Source: CAD feature listing. Evaluate the final solid. Frame: model axes, mm. A direction names the side the tool comes from. Round coordinates to 2 decimals unless told otherwise and drop trailing zeros. Order: outer loops, then holes, each group sorted by start corner. A loop starts at its lowest first (then second) coordinate and runs counter-clockwise, first axis right, second up. Notation, with made-up numbers: (61, 83) -> (92, 83) arc R18 cw to (92, 108) -> close; hole circle Ø4 at (88, 20). An arc over 180 degrees is marked (long way). Use a Markdown table: item, result. Add a question column.
```python
from build123d import *

# Parameters (mm, degrees)
AUFSATZ_LINEAR_AUSTRAGEN1_DEPTH             = 20
AUFSATZ_LINEAR_AUSTRAGEN2_REACH             = 50.332
AUFSATZ_LINEAR_AUSTRAGEN2_DIRECTION_2_REACH = 50.332
SKIZZE2_R                                   = 2.3
SCHNITT_LINEAR_AUSTRAGEN1_DEPTH             = 20
SKIZZE4_R                                   = 4.2
SCHNITT_LINEAR_AUSTRAGEN2_DEPTH             = 20
VERRUNDUNG1_R                               = 0.75
VERRUNDUNG2_R                               = 4
SKIZZE5_R                                   = 1.7499999999999998
SCHNITT_LINEAR_AUSTRAGEN3_DEPTH             = 20
FASE1_SIZE                                  = 0.5


with BuildPart() as part:
    # Skizze1 → Aufsatz-Linear austragen1 (new body)
    with BuildSketch(Plane.XY):
        Polygon((-11, 0), (11, 0), (21.999999999999947, 19.052558883257674), (10.999999999999858, 38.10511776651528), (-10.999999999999858, 38.10511776651528), (-21.999999999999947, 19.052558883257674), align=None)
        Polygon((0, 7), (6.958548115672608, 7), (13.917096231345187, 19.052558883257657), (6.958548115672503, 31.105117766515278), (-6.958548115672498, 31.105117766515278), (-13.917096231345184, 19.05255888325765), (-6.958548115672604, 7), align=None, mode=Mode.SUBTRACT)
    extrude(amount=AUFSATZ_LINEAR_AUSTRAGEN1_DEPTH)

    # Aufsatz-Linear austragen2: up to this plane
    aufsatz_linear_austragen2_end = Plane(origin=(11, 0, 20), z_dir=(-0.86602540378444, 0.4999999999999978, 0))
    # Skizze3 → Aufsatz-Linear austragen2 (add, up to the surface)
    with BuildSketch(Plane(origin=(0, 0, 0), x_dir=(0, 0, -1), z_dir=(1, 0, 0)), mode=Mode.PRIVATE) as aufsatz_linear_austragen2_sk1:
        Polygon((-13.5, 8.3e-16), (-6.500000000000001, 8.3e-16), (-7.250000000000007, -0.7499999999999989), (-12.749999999999995, -0.7499999999999989), align=None)
    aufsatz_linear_austragen2_tool1 = split(extrude(aufsatz_linear_austragen2_sk1.sketch, amount=AUFSATZ_LINEAR_AUSTRAGEN2_REACH, mode=Mode.PRIVATE), bisect_by=aufsatz_linear_austragen2_end, keep=Keep.BOTH, mode=Mode.PRIVATE)
    add(aufsatz_linear_austragen2_tool1.solids().sort_by_distance((0, -0.36, 10))[0])

    # Aufsatz-Linear austragen2 direction 2: up to this plane
    aufsatz_linear_austragen2_direction_2_end = Plane(origin=(-11, 0, 20), z_dir=(0.86602540378444, 0.4999999999999978, 0))
    # Skizze3 → Aufsatz-Linear austragen2 direction 2 (add, up to the surface)
    with BuildSketch(Plane(origin=(0, 0, 0), x_dir=(0, 0, -1), z_dir=(1, 0, 0)), mode=Mode.PRIVATE) as aufsatz_linear_austragen2_direction_2_sk1:
        Polygon((-13.5, 8.3e-16), (-6.500000000000001, 8.3e-16), (-7.250000000000007, -0.7499999999999989), (-12.749999999999995, -0.7499999999999989), align=None)
    aufsatz_linear_austragen2_direction_2_tool1 = split(extrude(aufsatz_linear_austragen2_direction_2_sk1.sketch, amount=-AUFSATZ_LINEAR_AUSTRAGEN2_DIRECTION_2_REACH, mode=Mode.PRIVATE), bisect_by=aufsatz_linear_austragen2_direction_2_end, keep=Keep.BOTH, mode=Mode.PRIVATE)
    add(aufsatz_linear_austragen2_direction_2_tool1.solids().sort_by_distance((0, -0.36, 10))[0])

    # Skizze2 → Schnitt-Linear austragen1 (cut)
    with BuildSketch(Plane(origin=(0, 7, 0), x_dir=(1, 0, 0), z_dir=(0, 1, 0))):
        with Locations(Location((6.94e-15, -10, 0), (0, 0, 270))):
            Circle(SKIZZE2_R)
    extrude(amount=-SCHNITT_LINEAR_AUSTRAGEN1_DEPTH, mode=Mode.SUBTRACT)

    # Skizze4 → Schnitt-Linear austragen2 (cut)
    with BuildSketch(Plane.XZ):
        with Locations((6.94e-15, 10)):
            Circle(SKIZZE4_R)
    extrude(amount=SCHNITT_LINEAR_AUSTRAGEN2_DEPTH, mode=Mode.SUBTRACT)

    # Verrundung1
    verrundung1_edges = [part.edges().sort_by_distance(p)[0] for p in [
        (-4.199999999999993, -0.7499999999999989, 10),
        (4.200000000000008, -0.7499999999999989, 10),
    ]]
    fillet(verrundung1_edges, radius=VERRUNDUNG1_R - 0.0001)  # a hair under: the kernel refuses the full size

    # Verrundung2
    verrundung2_edges = [part.edges().sort_by_distance(p)[0] for p in [
        (11, 0, 16.75),
        (-11, 0, 16.75),
        (-21.999999999999947, 19.052558883257674, 10),
        (-10.999999999999858, 38.10511776651528, 10),
        (10.999999999999858, 38.10511776651528, 10),
        (21.999999999999947, 19.052558883257674, 10),
        (-6.958548115672604, 7, 10),
        (6.958548115672608, 7, 10),
        (13.917096231345187, 19.052558883257657, 10),
        (6.958548115672503, 31.105117766515278, 10),
        (-6.958548115672498, 31.105117766515278, 10),
        (-13.917096231345184, 19.05255888325765, 10),
        (11, 0, 3.2500000000000004),
        (-11, 0, 3.2500000000000004),
        (10.783493649053893, -0.3750000000000009, 6.875000000000002),
        (10.566987298107785, -0.749999999999999, 10),
        (10.783493649053893, -0.37499999999999845, 13.124999999999996),
        (-10.783493649053893, -0.37499999999999845, 13.124999999999996),
        (-10.783493649053893, -0.3750000000000009, 6.875000000000002),
        (-10.566987298107785, -0.749999999999999, 10),
    ]]
    fillet(verrundung2_edges, radius=VERRUNDUNG2_R)

    # Skizze5 → Schnitt-Linear austragen3 (cut)
    with BuildSketch(Plane.XZ.offset(-31.105117766515278)):
        with Locations(Location((6.94e-15, 10, 0), (0, 0, 270))):
            Circle(SKIZZE5_R)
    extrude(amount=-SCHNITT_LINEAR_AUSTRAGEN3_DEPTH, mode=Mode.SUBTRACT)

    # Fase1
    fase1_edges = [part.edges().sort_by_distance(p)[0] for p in [
        (-10.437822173508891, 13.026279441628823, 0),
        (-21.38119784648294, 19.052558883257667, 0),
        (-10.69059892324136, 37.569219381653035, 0),
        (10.69059892324136, 37.569219381653035, 0),
        (21.38119784648294, 19.052558883257674, 0),
        (-10.690598923241494, 0.5358983848622438, 0),
        (10.690598923241497, 0.5358983848622478, 0),
        (1.78e-15, 0, 20),
        (16.4999999999999, 28.578838324886483, 20),
        (0, 38.10511776651528, 20),
        (-16.4999999999999, 28.57883832488648, 20),
        (-16.49999999999997, 9.526279441628835, 20),
        (10.437822173508899, 13.02627944162883, 20),
        (8.9e-16, 7, 20),
        (-10.437822173508891, 13.026279441628823, 20),
        (-10.437822173508836, 25.078838324886473, 20),
        (2.66e-15, 31.105117766515278, 20),
        (10.437822173508838, 25.078838324886476, 20),
        (-21.38119784648294, 19.052558883257667, 20),
        (-10.69059892324136, 37.569219381653035, 20),
        (10.69059892324136, 37.569219381653035, 20),
        (21.38119784648294, 19.052558883257674, 20),
        (-10.690598923241494, 0.5358983848622438, 20),
        (10.690598923241497, 0.5358983848622478, 20),
        (13.298294077828178, 19.05255888325766, 0),
        (13.298294077828178, 19.05255888325766, 20),
        (6.649147038914101, 7.535898384862248, 0),
        (6.649147038914101, 7.535898384862248, 20),
        (-6.6491470389141, 7.5358983848622465, 0),
        (-6.6491470389141, 7.5358983848622465, 20),
        (-13.298294077828174, 19.052558883257642, 0),
        (-13.298294077828174, 19.052558883257642, 20),
        (-6.649147038914, 30.56921938165304, 0),
        (-6.649147038914, 30.56921938165304, 20),
        (6.649147038914005, 30.56921938165304, 0),
        (6.649147038914005, 30.56921938165304, 20),
        (7.47e-15, 38.10511776651528, 11.75),
        (7.47e-15, 31.105117766515278, 11.75),
        (7.64e-15, 7, 7.7),
        (7.64e-15, 0, 7.7),
        (16.499999999999975, 9.526279441628839, 0),
        (16.499999999999975, 9.526279441628839, 20),
        (1.78e-15, 0, 0),
        (-16.49999999999997, 9.526279441628835, 0),
        (-16.4999999999999, 28.57883832488648, 0),
        (0, 38.10511776651528, 0),
        (16.4999999999999, 28.578838324886483, 0),
        (0, 7, 0),
        (10.437822173508899, 13.02627944162883, 0),
        (10.437822173508838, 25.078838324886476, 0),
        (2.66e-15, 31.105117766515278, 0),
        (-10.437822173508836, 25.078838324886473, 0),
    ]]
    chamfer(fase1_edges, length=FASE1_SIZE)


solid = part.part
```
1) Draft query along X for faces 4 (the cylindrical face through (-9.87, -0.41, 9.96)), 5 (the flat face through (7, -0.75, 10)), 6 (the cylindrical face through (0.526, 34.563, 8.331)). Return one class per face: pulls with the +X half, pulls with the -X half, needs draft (parallel to the pull), parting line crosses it, or undercut.
2) Section D-D on x = 18. Output: boundary loops of the cut face in (y, z), then the cut area to 3 significant figures.
3) Section B-B on x = 0. Count the separate pieces of the cut face and the enclosed holes in it, then the cut area to 3 significant figures.
4) First-contact query: pin 1 Ø8 at (y, z) = (25.5, 5) entering from -X; pin 2 Ø3 at (x, z) = (0, 10) entering from +Y; pin 3 Ø2 at (x, z) = (17, 13) entering from +Y; pin 4 Ø3 at (x, z) = (-0.5, 6) entering from -Y. Flat tips, straight axial feed; report the tip coordinate or a pass-through.
5) Line query: probe 1 along Y at (x, z) = (1.5, 18); probe 2 along X at (y, z) = (9.5, 8.5); probe 3 along X at (y, z) = (35.3, 10). Output: solid intervals per line, ascending. Write a range as from..to.
6) Section C-C on y = 9.5. Output: boundary loops of the cut face in (x, z), then the cut area to 3 significant figures.
7) Reachability of faces 1 (the cylindrical face through (0.101, 3.542, 7.702)), 2 (the flat face through (10.619, 12.847, 19.746)), 3 (the flat face through (10.47, 25.02, 9.87)) from +Z, -Z, +X, -X, +Y, -Y: full face, straight path, thin tool, end or side. Return the list, or none.
8) Section A-A on z = 2.75. Output: boundary loops of the cut face in (x, y).
Conclusion:
| question | item | result |
|---|---|---|
| 1 | face 4 | pulls with the -X half |
| 1 | face 5 | needs draft |
| 1 | face 6 | undercut |
| 2 | outline | (12.12, 0.5) -> (13.12, 0) -> (24.98, 0) -> (25.98, 0.5) -> (25.98, 19.5) -> (24.98, 20) -> (13.12, 20) -> (12.12, 19.5) -> close |
| 2 | area | 276 mm^2 |
| 3 | separate pieces | 4 |
| 3 | enclosed holes | 0 |
| 3 | area | 221 mm^2 |
| 4 | pin 1 | stops at x = -20.59 |
| 4 | pin 2 | passes through |
| 4 | pin 3 | stops at y = 29.44 |
| 4 | pin 4 | stops at y = 0 |
| 5 | probe 1 | y = 0..7, 31.11..38.11 |
| 5 | probe 2 | x = -16.48..-8.4, 8.4..16.48 |
| 5 | probe 3 | x = -12.62..-1.75, 1.75..12.62 |
| 6 | outline | (-16.48, 0.5) -> (-15.91, 0) -> (-8.98, 0) -> (-8.4, 0.5) -> (-8.4, 19.5) -> (-8.98, 20) -> (-15.91, 20) -> (-16.48, 19.5) -> close; (8.4, 0.5) -> (8.98, 0) -> (15.91, 0) -> (16.48, 0.5) -> (16.48, 19.5) -> (15.91, 20) -> (8.98, 20) -> (8.4, 19.5) -> close |
| 6 | area | 322 mm^2 |
| 7 | face 1 | -Y |
| 7 | face 2 | +Z |
| 7 | face 3 | +Z, -Z |
| 8 | outline | (-20.85, 17.05) -> (-12.15, 2) arc R4 ccw to (-8.69, 0) -> (8.69, 0) arc R4 ccw to (12.15, 2) -> (20.85, 17.05) arc R4 ccw to (20.85, 21.05) -> (12.15, 36.11) arc R4 ccw to (8.69, 38.11) -> (-8.69, 38.11) arc R4 ccw to (-12.15, 36.11) -> (-20.85, 21.05) arc R4 ccw to start; hole (-12.76, 17.05) -> (-8.11, 9) arc R4 ccw to (-4.65, 7) -> (4.65, 7) arc R4 ccw to (8.11, 9) -> (12.76, 17.05) arc R4 ccw to (12.76, 21.05) -> (8.11, 29.11) arc R4 ccw to (4.65, 31.11) -> (-4.65, 31.11) arc R4 ccw to (-8.11, 29.11) -> (-12.76, 21.05) arc R4 ccw to start |
